Could you check a few things on this model? Use its own coordinates, in mm. A direction names the side the tool comes from. Give positions to 0.01 mm unless a question says otherwise; leave off trailing zeros. Order: outer loops, then holes, each group sorted by start corner. A loop starts at its lowest first (then second) coordinate and runs counter-clockwise, first axis right, second up.
(1) On a 3-axis mill with a long thin cutter (end or side, diameter ignored), from which of +Z, -Z, +X, -X, +Y, -Y can I reach the whole of each face in a straight line? I mean faces 1 (the flat face through (-20, 7.5, 10)), 2 (the flat face through (13.38, 14.92, 5.44)), 3 (the cylindrical face through (1.14, 4.51, 8.73)). Say none if no direction works.
(2) If we mould it in two halves opening along X, with no side actions, what happens to faces 4 (the flat face through (12, 0, 12.65)), 5 (the cylindrical face through (-4.83, 10.63, 11.43)), 6 (the flat face through (-13, -14, 10))? For each: released by +X, released by -X, zero draft, split by the parting line, or undercut.
(3) Imagine slicing it at C-C, the plane x = -27. Write out the boundary of the cut face in (y, z), then the cut area to 3 significant figures.
(4) Will these pins go through, and if not, where does the flat tip stop? pin 1 (2.5 mm diameter, centred on x = 12.5, y = 10, fed in from -Z); pin 2 (1.6 mm diameter, centred on y = -9.5, z = 1, fed in from -X); pin 3 (6 mm diameter, centred on x = 30.5, z = 10.5, fed in from +Y).
(5) If I drill on probe 1 along Y at (x, z) = (30.5, 1.75); probe 2 along Y at (x, z) = (-17, 2.75); probe 3 along Y at (x, z) = (-9, 2.5), over which ranges is the centre line in solid material (lowest first)?
(6) Imagine slicing it at A-A, the plane y = 0. Write out the boundary of the cut face in (x, z).
(7) Imagine slicing it at B-B, the plane x = 29. Write out the boundary of the cut face in (y, z), then the cut area to 3 significant figures.
(8) Imagine slicing it at D-D, the plane z = 2. State how many separate pieces and enclosed holes the cut face has, then the cut area to 3 significant figures.
from build123d import *

# Parameters (mm, degrees)
BOSS_EXTRUDE1_DEPTH             = 12.65
CUT_EXTRUDE1_START              = -5.5
CUT_EXTRUDE1_DEPTH              = 5.5
CUT_EXTRUDE3_DEPTH              = 40.349364671
CUT_EXTRUDE4_DEPTH              = 58
CUT_EXTRUDE5_DEPTH              = 3.25
CUT_EXTRUDE6_DEPTH              = 7.25
M10_CLEARANCE_HOLE1_D           = 10.5
CBORE_START                     = 7.25
CBORE_SLOT_FOR_M3_SHCS1_DEPTH   = 3
CBORE_START_2                   = 10.25
CBORE_SLOT_FOR_M3_SHCS1_2_DEPTH = 2.4
CIRPATTERN1_COUNT               = 4
M4_CLEARANCE_HOLE1_D            = 4.5
BOSS_EXTRUDE2_START             = 4
BOSS_EXTRUDE2_DEPTH             = 4
CUT_EXTRUDE7_DEPTH              = 3.2
FILLET1_R                       = 1
FILLET1_OF_MIRROR1_R            = 1


# Read off the part's stored shape, not the designer's step: CBORE SLOT for M3 SHCS1
with BuildPart() as part:
    # Sketch2 → Boss-Extrude1 (new body)
    with BuildSketch(Plane.XY):
        with BuildLine():
            Line((32, 16.5), (-30, 16.5))
            ThreePointArc((-30, 16.5), (-33.535533906, 15.035533906), (-35, 11.5))
            Line((-35, 11.5), (-35, -11.5))
            ThreePointArc((-35, -11.5), (-33.535533906, -15.035533906), (-30, -16.5))
            Line((-30, -16.5), (32, -16.5))
            ThreePointArc((32, -16.5), (34.121320344, -15.621320344), (35, -13.5))
            Line((35, -13.5), (35, 13.5))
            ThreePointArc((35, 13.5), (34.121320344, 15.621320344), (32, 16.5))
        make_face()
    extrude(amount=BOSS_EXTRUDE1_DEPTH)

    # Sketch3 → Cut-Extrude1 (cut)
    with BuildSketch(Plane.XY.offset(12.65).offset(CUT_EXTRUDE1_START)):
        with BuildLine():
            Line((-13, 10.5), (-13, 16.5))
            Line((-13, 16.5), (-30, 16.5))
            ThreePointArc((-30, 16.5), (-33.535533906, 15.035533906), (-35, 11.5))
            Line((-35, 11.5), (-35, -11.5))
            ThreePointArc((-35, -11.5), (-33.535533906, -15.035533906), (-30, -16.5))
            Line((-30, -16.5), (-13, -16.5))
            Line((-13, -16.5), (-13, -10.5))
            ThreePointArc((-13, -10.5), (-13.878679656, -8.378679656), (-16, -7.5))
            Line((-16, -7.5), (-23, -7.5))
            Line((-23, -7.5), (-23, 7.5))
            Line((-23, 7.5), (-16, 7.5))
            ThreePointArc((-16, 7.5), (-13.878679656, 8.378679656), (-13, 10.5))
        make_face()
        with BuildLine():
            Line((32, 16.5), (24.5, 16.5))
            Line((24.5, 16.5), (24.5, 10.5))
            ThreePointArc((24.5, 10.5), (25.378679656, 8.378679656), (27.5, 7.5))
            Line((27.5, 7.5), (35, 7.5))
            Line((35, 7.5), (35, 13.5))
            ThreePointArc((35, 13.5), (34.121320344, 15.621320344), (32, 16.5))
        make_face()
        with BuildLine():
            Line((35, -13.5), (35, -7.5))
            Line((35, -7.5), (27.5, -7.5))
            ThreePointArc((27.5, -7.5), (25.378679656, -8.378679656), (24.5, -10.5))
            Line((24.5, -10.5), (24.5, -16.5))
            Line((24.5, -16.5), (32, -16.5))
            ThreePointArc((32, -16.5), (34.121320344, -15.621320344), (35, -13.5))
        make_face()
    extrude(amount=CUT_EXTRUDE1_DEPTH, mode=Mode.SUBTRACT)

    # Sketch5 → Cut-Extrude3 (cut, through all)
    with BuildSketch(Plane.XY.offset(7.15)):
        with BuildLine():
            Line((-23, -5.5), (-24.995769837, -5.5))
            ThreePointArc((-24.995769837, -5.5), (-25.705460123, -5.793963342), (-25.999423465, -6.503653628))
            ThreePointArc((-25.999423465, -6.503653628), (-28.999423465, -9.503653628), (-31.999423465, -6.503653628))
            Line((-31.999423465, -6.503653628), (-31.999423465, 6.503653628))
            ThreePointArc((-31.999423465, 6.503653628), (-28.999423465, 9.503653628), (-25.999423465, 6.503653628))
            ThreePointArc((-25.999423465, 6.503653628), (-25.705460123, 5.793963342), (-24.995769837, 5.5))
            Line((-24.995769837, 5.5), (-23, 5.5))
            Line((-23, 5.5), (-23, -5.5))
        make_face()
    extrude(amount=-CUT_EXTRUDE3_DEPTH, mode=Mode.SUBTRACT)

    # Sketch4 → Cut-Extrude4 (cut)
    with BuildSketch(Plane(origin=(35, 0, 0), x_dir=(0, 0, -1), z_dir=(1, 0, 0))):
        with BuildLine():
            Line((0, -8), (0, 8))
            ThreePointArc((0, 8), (-8, 0), (0, -8))
        make_face()
    extrude(amount=-CUT_EXTRUDE4_DEPTH, mode=Mode.SUBTRACT)

    # Sketch6 → Cut-Extrude5 (cut)
    with BuildSketch(Plane(origin=(0, 0, 0), x_dir=(-1, 0, 0), z_dir=(0, 0, -1))):
        with BuildLine():
            Line((30, -16.5), (20, -16.5))
            ThreePointArc((20, -16.5), (22.121320344, -15.621320344), (23, -13.5))
            Line((23, -13.5), (23, 13.5))
            ThreePointArc((23, 13.5), (22.121320344, 15.621320344), (20, 16.5))
            Line((20, 16.5), (30, 16.5))
            ThreePointArc((30, 16.5), (33.535533906, 15.035533906), (35, 11.5))
            Line((35, 11.5), (35, -11.5))
            ThreePointArc((35, -11.5), (33.535533906, -15.035533906), (30, -16.5))
        make_face()
    extrude(amount=-CUT_EXTRUDE5_DEPTH, mode=Mode.SUBTRACT)

    # Sketch7 → Cut-Extrude6 (cut)
    with BuildSketch(Plane(origin=(0, 0, 0), x_dir=(-1, 0, 0), z_dir=(0, 0, -1))):
        with BuildLine():
            Line((9.5, -13.3), (-21.5, -13.3))
            ThreePointArc((-21.5, -13.3), (-22.914213562, -12.714213562), (-23.5, -11.3))
            Line((-23.5, -11.3), (-23.5, 11.3))
            ThreePointArc((-23.5, 11.3), (-22.914213562, 12.714213562), (-21.5, 13.3))
            Line((-21.5, 13.3), (9.5, 13.3))
            ThreePointArc((9.5, 13.3), (10.914213562, 12.714213562), (11.5, 11.3))
            Line((11.5, 11.3), (11.5, -11.3))
            ThreePointArc((11.5, -11.3), (10.914213562, -12.714213562), (9.5, -13.3))
        make_face()
    extrude(amount=-CUT_EXTRUDE6_DEPTH, mode=Mode.SUBTRACT)

    # M10 Clearance Hole1 (through all)
    with Locations(Plane.XY.offset(12.65)):
        with Locations((5.75, 0)):
            Hole(M10_CLEARANCE_HOLE1_D / 2)

    # CBORE SLOT for M3 SHCS1 outline → CBORE SLOT for M3 SHCS1 (cut)
    with BuildSketch(Plane.XY.offset(CBORE_START)):
        with BuildLine():
            ThreePointArc((12.856423151, -11.702617229), (17.452617229, -11.702617229), (17.452617229, -7.106423151))
            Line((17.452617229, -7.106423151), (14.907032816, -4.560838739))
            ThreePointArc((14.907032816, -4.560838739), (10.310838739, -4.560838739), (10.310838739, -9.157032816))
            Line((10.310838739, -9.157032816), (12.856423151, -11.702617229))
        make_face()
    cbore_slot_for_m3_shcs1 = extrude(amount=CBORE_SLOT_FOR_M3_SHCS1_DEPTH, mode=Mode.SUBTRACT)

    # CBORE SLOT for M3 SHCS1 2 outline → CBORE SLOT for M3 SHCS1 2 (cut)
    with BuildSketch(Plane.XY.offset(CBORE_START_2)):
        with BuildLine():
            ThreePointArc((13.952438662, -10.606601718), (16.356601718, -10.606601718), (16.356601718, -8.202438662))
            Line((16.356601718, -8.202438662), (13.811017306, -5.656854249))
            ThreePointArc((13.811017306, -5.656854249), (11.406854249, -5.656854249), (11.406854249, -8.061017306))
            Line((11.406854249, -8.061017306), (13.952438662, -10.606601718))
        make_face()
    cbore_slot_for_m3_shcs1_2 = extrude(amount=CBORE_SLOT_FOR_M3_SHCS1_2_DEPTH, mode=Mode.SUBTRACT)

    # CirPattern1: CBORE SLOT for M3 SHCS1, CBORE SLOT for M3 SHCS1 2 ×4 about axis
    cirpattern1_axis = Axis((5.75, 0, 0), (0, 0, 1))
    add([cbore_slot_for_m3_shcs1.rotate(cirpattern1_axis, i * 360 / CIRPATTERN1_COUNT) for i in range(1, CIRPATTERN1_COUNT)], mode=Mode.SUBTRACT)
    add([cbore_slot_for_m3_shcs1_2.rotate(cirpattern1_axis, i * 360 / CIRPATTERN1_COUNT) for i in range(1, CIRPATTERN1_COUNT)], mode=Mode.SUBTRACT)

    # M4 Clearance Hole1 (through all)
    with Locations(Plane.XY.offset(7.15)):
        with Locations((29, -11.5), (29, 11.5), (-17, 11.5), (-17, -11.5)):
            Hole(M4_CLEARANCE_HOLE1_D / 2)

    # Sketch19 → Boss-Extrude2 (add)
    with BuildSketch(Plane(origin=(-23, 0, 0), x_dir=(0, 0, -1), z_dir=(1, 0, 0)).offset(BOSS_EXTRUDE2_START)):
        with BuildLine():
            Line((-3.25, 5.5), (-3.25, 7.310095759))
            ThreePointArc((-3.25, 7.310095759), (-4.619267644, 6.531643471), (-5.809475019, 5.5))
            Line((-5.809475019, 5.5), (-3.25, 5.5))
        make_face()
        with BuildLine():
            Line((-3.25, -7.310095759), (-3.25, -5.5))
            Line((-3.25, -5.5), (-5.809475019, -5.5))
            ThreePointArc((-5.809475019, -5.5), (-4.619267644, -6.531643471), (-3.25, -7.310095759))
        make_face()
    extrude(amount=-BOSS_EXTRUDE2_DEPTH)

    # Sketch20 → Cut-Extrude7 (cut)
    with BuildSketch(Plane(origin=(0, 16.5, 0), x_dir=(1, 0, 0), z_dir=(0, 1, 0))):
        Polygon((-2.5, 0), (14, 0), (12.75, -11), (-1.25, -11), align=None)
    cut_extrude7 = extrude(amount=-CUT_EXTRUDE7_DEPTH, mode=Mode.SUBTRACT)

    # Fillet1
    fillet1_edges = [part.edges().sort_by_distance(p)[0] for p in [
        (-1.25, 14.9, 11),
        (-2.5, 14.9, 0),
        (14, 14.9, 0),
        (12.75, 14.9, 11),
    ]]
    fillet(fillet1_edges, radius=FILLET1_R)

    # Mirror1: Cut-Extrude7 across plane
    add(cut_extrude7.mirror(Plane.ZX), mode=Mode.SUBTRACT)

    # Fillet1 of Mirror1
    fillet1_of_mirror1_edges = [part.edges().sort_by_distance(p)[0] for p in [
        (-1.25, -14.9, 11),
        (-2.5, -14.9, 0),
        (14, -14.9, 0),
        (12.75, -14.9, 11),
    ]]
    fillet(fillet1_of_mirror1_edges, radius=FILLET1_OF_MIRROR1_R)


solid = part.part
Answer block:
1. face 1: +Z, -X, +Y
1. face 2: -Z, +Y
1. face 3: -Z
2. face 4: zero draft
2. face 5: undercut
2. face 6: released by -X
3. outline: (-16.5, 3.25) - (-8.74, 3.25) - (-8.74, 7.15) - (-16.5, 7.15) - close; (8.74, 3.25) - (16.5, 3.25) - (16.5, 7.15) - (8.74, 7.15) - close
3. area: 60.5 mm2
4. pin 1: stops at z = 7.25
4. pin 2: stops at x = -23
4. pin 3: stops at y = 7.5
5. probe 1: y = -16.5 to -13.18, -9.82 to -7.81, 7.81 to 9.82, 13.18 to 16.5
5. probe 2: y = -16.5 to -13.75, -9.25 to -7.51, 7.51 to 9.25, 13.75 to 16.5
5. probe 3: y = -16.5 to -13.3, 13.3 to 16.5
6. outline: (-35, 3.25) - (-32, 3.25) - (-32, 7.15) - (-35, 7.15) - close; (-23, 8) - (0.5, 8) - (0.5, 12.65) - (-23, 12.65) - close; (11, 8) - (35, 8) - (35, 12.65) - (11, 12.65) - close
7. outline: (-16.5, 0) - (-13.75, 0) - (-13.75, 7.15) - (-16.5, 7.15) - close; (-9.25, 0) - (-8, 0) arc R8 cw to (8, 0) - (9.25, 0) - (9.25, 7.15) - (7.5, 7.15) - (7.5, 12.65) - (-7.5, 12.65) - (-7.5, 7.15) - (-9.25, 7.15) - close; (13.75, 0) - (16.5, 0) - (16.5, 7.15) - (13.75, 7.15) - close
7. area: 154 mm2
8. separate pieces: 4
8. enclosed holes: 4
8. area: 456 mm2
